Could you check a few things on this model? Use its own coordinates, in mm. Face numbers are marked on the shaded views. A direction names the side the tool comes from. Round coordinates to 2 decimals unless told otherwise and drop trailing zeros. Loops run counter-clockwise (first coordinate to the right, second up) from the corner with the lowest first, then second, coordinate; pieces in that order, holes last. Notation, with made-up numbers: M 45,26.25 L 52,26.25 A30 ccw 52,64.25 Z; hole C 23,1.25 d11. An arc over 180 degrees is marked long. One line per item, written item: value. Start each with the question number.
Q1. Thinking about a two-plate mould opening in X: for the marked faces 4, 5 and 6, which applies, released by +X, released by -X, zero draft, split by the parting line, or undercut?
Q2. Imagine slicing it at D-D (z = -20). Please give me the cut outline in (x, y).
Q3. Which directions (+Z, -Z, +X, -X, +Y, -Y) give clear straight access to the entire face, cutting with the end or side of a thin tool? Please do the marked faces 1, 2 and 3.
Q4. I'm going to push flat-ended pins straight in: pin 1 Ø3.5 at (y, z) = (11.5, -4) entering from +X; pin 2 Ø5 at (y, z) = (10.5, -14) entering from +X; pin 3 Ø5 at (x, y) = (13, 17) entering from +Z. Where does each tip first touch, or does it pass through?
Q5. Please list where these lines run through material, in increasing order: line 1 along Y through (x, z) = (13, -26.05); line 2 along Y through (x, z) = (1.2, -5); line 3 along X through (y, z) = (17.25, -15.5).
Q6. Imagine slicing it at A-A (z = -5). Please give me the cut outline in (x, y).
Q7. Imagine slicing it at C-C (x = 5.5). Please give me the cut outline in (y, z).
Q8. Imagine slicing it at B-B (y = 17). Please give me the cut outline in (x, z), then the cut area to 3 significant figures.
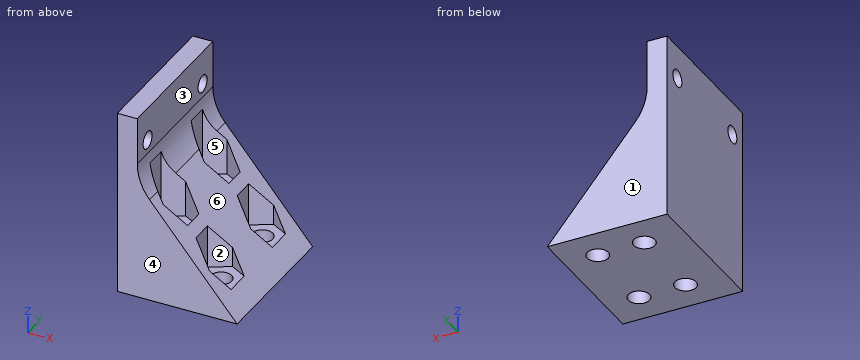
from build123d import *

# Parameters (mm, degrees)
SKETCH1_W           = 28
SKETCH1_H           = 22
SKETCH1_R           = 1.3
BOSS_EXTRUDE1_DEPTH = 3
BOSS_EXTRUDE3_DEPTH = 22
FILLET1_R           = 8
SKETCH4_R           = 1.6
CUT_EXTRUDE1_DEPTH  = 29
CUT_EXTRUDE2_DEPTH  = 20
CUT_EXTRUDE3_DEPTH  = 26


with BuildPart() as part:
    # Sketch1 → Boss-Extrude1 (new body)
    with BuildSketch(Plane(origin=(0, 0, 0), x_dir=(0, 0, -1), z_dir=(1, 0, 0))):
        with Locations((14, 11)):
            Rectangle(SKETCH1_W, SKETCH1_H)
        with Locations((5, 19)):
            Circle(SKETCH1_R, mode=Mode.SUBTRACT)
        with Locations((5, 3)):
            Circle(SKETCH1_R, mode=Mode.SUBTRACT)
    extrude(amount=BOSS_EXTRUDE1_DEPTH)

    # Sketch3 → Boss-Extrude3 (add)
    with BuildSketch(Plane(origin=(0, 0, 0), x_dir=(1, 0, 0), z_dir=(0, 1, 0))):
        Polygon((3, 28), (18, 28), (3, 10), align=None)
    extrude(amount=BOSS_EXTRUDE3_DEPTH)

    # Fillet1
    fillet1_edges = [part.edges().sort_by_distance(p)[0] for p in [
        (3, 11, -10),
    ]]
    fillet(fillet1_edges, radius=FILLET1_R)

    # Sketch4 → Cut-Extrude1 (cut, through all)
    with BuildSketch(Plane(origin=(0, 0, -28), x_dir=(-1, 0, 0), z_dir=(0, 0, -1))):
        with Locations((-6, 17)):
            Circle(SKETCH4_R)
        with Locations((-6, 5)):
            Circle(SKETCH4_R)
        with Locations((-13, 17)):
            Circle(SKETCH4_R)
        with Locations((-13, 5)):
            Circle(SKETCH4_R)
    extrude(amount=-CUT_EXTRUDE1_DEPTH, mode=Mode.SUBTRACT)

    # Sketch5 → Cut-Extrude2 (cut, through all)
    with BuildSketch(Plane.XY.offset(-19)):
        Polygon((3.169500163, 3.365810157), (3.169500163, 6.634189843), (6, 8.268379685), (8.830499837, 6.634189843), (8.830499837, 3.365810157), (6, 1.731620315), align=None)
        Polygon((3.169500163, 15.365810157), (6, 13.731620315), (8.830499837, 15.365810157), (8.830499837, 18.634189843), (6, 20.268379685), (3.169500163, 18.634189843), align=None)
    extrude(amount=CUT_EXTRUDE2_DEPTH, mode=Mode.SUBTRACT)

    # Sketch6 → Cut-Extrude3 (cut, through all)
    with BuildSketch(Plane.XY.offset(-25)):
        Polygon((10.1, 15.325684219), (13, 13.651368439), (15.9, 15.325684219), (15.9, 18.674315781), (13, 20.348631561), (10.1, 18.674315781), align=None)
        Polygon((10.1, 3.325684219), (10.1, 6.674315781), (13, 8.348631561), (15.9, 6.674315781), (15.9, 3.325684219), (13, 1.651368439), align=None)
    extrude(amount=CUT_EXTRUDE3_DEPTH, mode=Mode.SUBTRACT)


solid = part.part
Report:
1. face 4: zero draft
1. face 5: undercut
1. face 6: released by +X
2. outline: M 0,0 L 11.33,0 L 11.33,2.61 L 10.1,3.33 L 10.1,6.67 L 11.33,7.39 L 11.33,14.61 L 10.1,15.33 L 10.1,18.67 L 11.33,19.39 L 11.33,22 L 0,22 Z; hole C 6,5 d3.2; hole C 6,17 d3.2
3. face 1: +Z, -Z, +X, -X, +Y
3. face 2: +Z
3. face 3: +Z, +X, +Y, -Y
4. pin 1: stops at x = 3
4. pin 2: stops at x = 8.42
4. pin 3: stops at z = -25
5. line 1: y = 0 to 3.4, 6.6 to 15.4, 18.6 to 22
5. line 2: y = 0 to 1.7, 4.3 to 17.7, 20.3 to 22
5. line 3: x = 0 to 3.17
6. outline: M 0,0 L 3,0 L 3,1.7 L 0,1.7 Z; M 0,4.3 L 3,4.3 L 3,17.7 L 0,17.7 Z; M 0,20.3 L 3,20.3 L 3,22 L 0,22 Z
7. outline: M 0,-28 L 3.48,-28 L 3.48,-19 L 2.02,-19 L 2.02,-13 L 0,-13 Z; M 6.52,-28 L 15.48,-28 L 15.48,-19 L 14.02,-19 L 14.02,-13 L 7.98,-13 L 7.98,-19 L 6.52,-19 Z; M 18.52,-28 L 22,-28 L 22,-13 L 19.98,-13 L 19.98,-19 L 18.52,-19 Z
8. outline: M 0,-28 L 4.4,-28 L 4.4,-19 L 3.17,-19 L 3.17,-8.74 A8 cw 3,-7.1 L 3,0 L 0,0 Z; M 7.6,-28 L 11.4,-28 L 11.4,-25 L 10.1,-25 L 10.1,-18.52 L 8.83,-17 L 8.83,-19 L 7.6,-19 Z; M 14.6,-28 L 18,-28 L 15.5,-25 L 14.6,-25 Z
8. area: 133 mm²
